Build history of the part. All positions in model axes, mm. Face numbers are marked on the shaded views. A direction names the side the tool comes from. Round coordinates to 2 decimals unless told otherwise and drop trailing zeros. Write item = value, one per line.
from build123d import *

# Parameters (mm, degrees)
F0_W     = 5.715
F0_H     = 1.5875
F0_W_2   = 3.7885198835
F1_DEPTH = 1.5875
F0_W_3   = 6.35
F0_H_2   = 3.175
F0_H_3   = 1.905
F2_DEPTH = 4.445
F3_DEPTH = 4.445
F4_DEPTH = 1.5875
F5_DEPTH = 1.5875
F6_DEPTH = 12.3825
F7_DEPTH = 3.175
F8_DEPTH = 3.81
F0_W_4   = 7.62
F0_H_4   = 7.62
F9_DEPTH = 3.175


with BuildPart() as f1:
    # F0 (on Top) → F1 (new body)
    with BuildSketch(Plane.XY):
        Polygon((-9.525, -17.4625), (-3.81, -17.4625), (-3.81, -14.2875), (-6.35, -14.2875), (-9.525, -14.2875), align=None)
        Polygon((3.8314801165, -14.2875), (6.35, -14.2875), (6.35, 6.7148534581), (-6.35, 6.7148534581), (-6.35, -14.2875), (-3.81, -14.2875), (-3.7885198835, -14.2875), (-3.7885198835, -9.2075), (-3.7885198835, -1.5875), (3.8314801165, -1.5875), (3.8314801165, -9.2075), align=None)
        Polygon((-9.525, 17.4625), (-9.525, 14.2875), (-6.35, 14.2875), (-3.175, 14.2875), (-3.175, 17.4625), align=None)
        Polygon((6.35, 14.2875), (9.525, 14.2875), (9.525, 17.4625), (3.175, 17.4625), (3.175, 14.2875), align=None)
        with Locations((6.6675, -16.66875)):
            Rectangle(F0_W, F0_H)
        with Locations((1.9157400582, -16.66875)):
            Rectangle(F0_W_2, F0_H)
        Polygon((3.81, -15.875), (9.525, -15.875), (9.525, -14.2875), (6.35, -14.2875), (3.8314801165, -14.2875), (3.81, -14.2875), align=None)
        Polygon((-3.81, -17.4625), (0.0214801165, -17.4625), (0.0214801165, -15.875), (0.0214801165, -14.2875), (-3.7885198835, -14.2875), (-3.81, -14.2875), align=None)
        with Locations((1.9157400582, -15.08125)):
            Rectangle(F0_W_2, F0_H)
        Polygon((0.0214801165, -14.2875), (3.81, -14.2875), (3.8314801165, -14.2875), (3.8314801165, -9.2075), (-3.7885198835, -9.2075), (-3.7885198835, -14.2875), align=None)
        Polygon((1.9264801165, -13.0175), (0.0214801165, -13.0175), (-1.8835198835, -13.0175), (-1.8835198835, -10.4775), (1.9264801165, -10.4775), align=None, mode=Mode.SUBTRACT)
        Polygon((6.35, 6.7148534581), (6.35, 14.2875), (3.175, 14.2875), (3.175, 12.3825), (-3.175, 12.3825), (-3.175, 14.2875), (-6.35, 14.2875), (-6.35, 6.7148534581), align=None)
    extrude(amount=F1_DEPTH)

    # F0 (on Top) → F2 (join)
    with BuildSketch(Plane.XY):
        with Locations((0, 15.875)):
            Rectangle(F0_W_3, F0_H_2)
        with Locations((0, 13.335)):
            Rectangle(F0_W_3, F0_H_3)
    extrude(amount=F2_DEPTH)

    # F0 (on Top) → F3 (join)
    with BuildSketch(Plane.XY):
        with Locations((0, 18.25625)):
            Rectangle(F0_W_3, F0_H)
    extrude(amount=F3_DEPTH)

    # F0 (on Top) → F4 (cut)
    with BuildSketch(Plane.XY):
        with Locations((0, 18.25625)):
            Rectangle(F0_W_3, F0_H)
    extrude(amount=F4_DEPTH, mode=Mode.SUBTRACT)

    # F0 (on Top) → F5 (join)
    with BuildSketch(Plane.XY):
        Polygon((-9.525, 14.2875), (-9.525, -14.2875), (-6.35, -14.2875), (-6.35, 6.7148534581), (-6.35, 14.2875), align=None)
        Polygon((6.35, -14.2875), (9.525, -14.2875), (9.525, 14.2875), (6.35, 14.2875), (6.35, 6.7148534581), align=None)
    extrude(amount=F5_DEPTH)

    # F0 (on Top) → F6 (join)
    with BuildSketch(Plane.XY):
        Polygon((6.35, -14.2875), (9.525, -14.2875), (9.525, 14.2875), (6.35, 14.2875), (6.35, 6.7148534581), align=None)
        Polygon((-9.525, 14.2875), (-9.525, -14.2875), (-6.35, -14.2875), (-6.35, 6.7148534581), (-6.35, 14.2875), align=None)
    extrude(amount=-F6_DEPTH)

    # F0 (on Top) → F7 (join)
    with BuildSketch(Plane.XY):
        Polygon((-1.8835198835, -13.0175), (0.0214801165, -13.0175), (1.9264801165, -13.0175), (1.9264801165, -10.4775), (-1.8835198835, -10.4775), align=None)
        Polygon((1.6089801165, -12.3825), (0.0214801165, -12.3825), (-1.5660198835, -12.3825), (-1.5660198835, -11.1125), (1.6089801165, -11.1125), align=None, mode=Mode.SUBTRACT)
    extrude(amount=F7_DEPTH)

    # F0 (on Top) → F8 (join)
    with BuildSketch(Plane.XY):
        Polygon((-1.5660198835, -12.3825), (0.0214801165, -12.3825), (1.6089801165, -12.3825), (1.6089801165, -11.1125), (-1.5660198835, -11.1125), align=None)
    extrude(amount=F8_DEPTH)

    # F0 (on Top) → F9 (join)
    with BuildSketch(Plane.XY):
        with Locations((0.0214801165, -5.3975)):
            Rectangle(F0_W_4, F0_H_4)
    extrude(amount=F9_DEPTH)


solid = f1.part
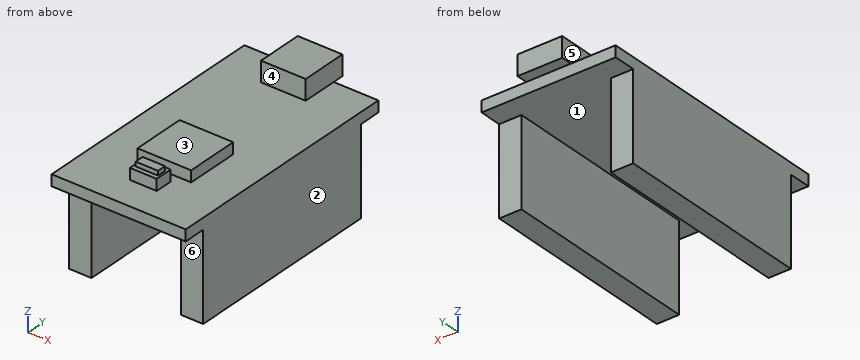
1. Mould opens along X. For the marked faces 1, 2 and 3 say: pulls with the +X half, pulls with the -X half, needs draft (parallel to the pull), parting line crosses it, or undercut.
Responses:
face_1 = undercut
face_2 = pulls with the +X half
face_3 = needs draft
2. Probe probe 1 along X at (y, z) = (-9, -9.75) (3 decimals); probe 2 along Z at (x, y) = (2.75, 13) (3 decimals); probe 3 along Z at (x, y) = (-2.5, -14.5). List the from-to ranges inside material, lowest first.
Responses:
probe_1 = -9.525 to -6.35, 6.35 to 9.525
probe_2 = 0 to 4.445
probe_3 = 0 to 1.59
3. Tool access for the marked faces 4, 5 and 6: list every direction of +Z, -Z, +X, -X, +Y, -Y with a clear straight run to the whole face (end or side of a thin tool).
Responses:
face_4 = +Z, +X, -X
face_5 = +Z, -X, +Y
face_6 = -Z, +X, -X, -Y
4. Flat gauge pins, fed straight in: pin 1 (3 mm diameter, centred on x = -7, z = -3, fed in from +Y); pin 2 (3 mm diameter, centred on y = 17, z = 3.5, fed in from -X) (3 decimals); pin 3 (1 mm diameter, centred on x = -7.5, z = -6.5, fed in from -Y); pin 4 (6 mm diameter, centred on x = 0.5, z = -4, fed in from +Y). Where does each tip first touch, or does it go through?
Responses:
pin_1 = 14.29
pin_2 = -3.175
pin_3 = -14.29
pin_4 = through
